CAD build for the part. Positions are in the model's coordinates, mm. A direction names the side the tool comes from. Round coordinates to 2 decimals unless told otherwise and drop trailing zeros. Write each loop counter-clockwise with the first axis right and the second up, starting at its lowest first coordinate (ties: lowest second). Pieces come first, ordered by that corner, then holes. Notation, with made-up numbers: (-1.5, 7) -> (37.5, 7) arc R25 cw to (37.5, 41) -> close; hole circle Ø7 at (89.25, -27). An arc over 180 degrees is marked (long way). Answer in a Markdown table with one row per item. Add a question column.
```python
from build123d import *

# Parameters (mm, degrees)
SKETCH1_R           = 16
SKETCH1_R_2         = 7
SKETCH1_R_3         = 1.5
BOSS_EXTRUDE1_DEPTH = 27.5
SKETCH1_3_R         = 9
SKETCH1_3_R_2       = 7
BOSS_EXTRUDE2_DEPTH = 29.5
SKETCH1_4_R         = 9
SKETCH1_4_R_2       = 7
BOSS_EXTRUDE3_DEPTH = 2


with BuildPart() as part:
    # Sketch1 → Boss-Extrude1 (new body)
    with BuildSketch(Plane.XY):
        Circle(SKETCH1_R)
        Circle(SKETCH1_R_2, mode=Mode.SUBTRACT)
        with Locations((-8.485281374, 8.485281374)):
            Circle(SKETCH1_R_3, mode=Mode.SUBTRACT)
        with Locations((8.485281374, 8.485281374)):
            Circle(SKETCH1_R_3, mode=Mode.SUBTRACT)
        with Locations((8.485281374, -8.485281374)):
            Circle(SKETCH1_R_3, mode=Mode.SUBTRACT)
        with Locations((-8.485281374, -8.485281374)):
            Circle(SKETCH1_R_3, mode=Mode.SUBTRACT)
    extrude(amount=BOSS_EXTRUDE1_DEPTH)

    # Sketch1_3 → Boss-Extrude2 (add)
    with BuildSketch(Plane.XY):
        Circle(SKETCH1_3_R)
        Circle(SKETCH1_3_R_2, mode=Mode.SUBTRACT)
    extrude(amount=BOSS_EXTRUDE2_DEPTH)

    # Sketch1_4 → Boss-Extrude3 (add)
    with BuildSketch(Plane.XY):
        Circle(SKETCH1_4_R)
        Circle(SKETCH1_4_R_2, mode=Mode.SUBTRACT)
    extrude(amount=-BOSS_EXTRUDE3_DEPTH)


solid = part.part
```
Item 1: Two-plate mould, pull along Y, no slides. Class faces 1 (the cylindrical face through (-7.68, 9.75, 13.56)), 2 (the flat face through (7, -7, 0)), 3 (the cylindrical face through (-1.172, 8.923, -0.986)): +Y half, -Y half, draft (parallel to the pull), parting line (faces both ways), or undercut.
Item 2: Saw through at C-C on y = 8. Give the cut face in (x, z).
Item 3: Saw through at B-B on x = 8.5. Give the cut face in (y, z), then the cut area to 3 significant figures.
Item 4: Saw through at A-A on y = 0. Give the cut face in (x, z), then the cut area to 3 significant figures.
Item 5: Drill centre lines: probe 1 along Y at (x, z) = (-0.5, 23); probe 2 along X at (y, z) = (9.5, 21); probe 3 along Z at (x, y) = (-10.5, -6.5). Where is each one in solid material? Low to high.
Item 6: Tool access for faces 4 (the flat face through (7, -7, 27.5)), 5 (the flat face through (0, -7.3, 29.5)): list every direction of +Z, -Z, +X, -X, +Y, -Y with a clear straight run to the whole face (end or side of a thin tool).
Item 7: Pin check, flat tips, straight feed: pin 1 (1.5 mm diameter, centred on x = 12.5, z = 7.5, fed in from +Y); pin 2 (2 mm diameter, centred on y = -8.5, z = 22.5, fed in from +X); pin 3 (1 mm diameter, centred on y = -10.5, z = 3, fed in from -X). Stop position of each tip, or through.
Recorded:
| question | item | result |
|---|---|---|
| 1 | face 1 | undercut |
| 1 | face 2 | draft |
| 1 | face 3 | parting line |
| 2 | outline | (-13.86, 0) -> (-9.9, 0) -> (-9.9, 27.5) -> (-13.86, 27.5) -> close; (-7.07, 0) -> (-4.12, 0) -> (-4.12, -2) -> (4.12, -2) -> (4.12, 0) -> (7.07, 0) -> (7.07, 27.5) -> (4.12, 27.5) -> (4.12, 29.5) -> (-4.12, 29.5) -> (-4.12, 27.5) -> (-7.07, 27.5) -> close; (9.9, 0) -> (13.86, 0) -> (13.86, 27.5) -> (9.9, 27.5) -> close |
| 3 | outline | (-13.56, 0) -> (-9.99, 0) -> (-9.99, 27.5) -> (-13.56, 27.5) -> close; (-6.99, 0) -> (-2.96, 0) -> (-2.96, -2) -> (2.96, -2) -> (2.96, 0) -> (6.99, 0) -> (6.99, 27.5) -> (2.96, 27.5) -> (2.96, 29.5) -> (-2.96, 29.5) -> (-2.96, 27.5) -> (-6.99, 27.5) -> close; (9.99, 0) -> (13.56, 0) -> (13.56, 27.5) -> (9.99, 27.5) -> close |
| 3 | area | 604 mm2 |
| 4 | outline | (-16, 0) -> (-9, 0) -> (-9, -2) -> (-7, -2) -> (-7, 29.5) -> (-9, 29.5) -> (-9, 27.5) -> (-16, 27.5) -> close; (7, -2) -> (9, -2) -> (9, 0) -> (16, 0) -> (16, 27.5) -> (9, 27.5) -> (9, 29.5) -> (7, 29.5) -> close |
| 4 | area | 511 mm2 |
| 5 | probe 1 | -15.99 to -6.98, 6.98 to 15.99 |
| 5 | probe 2 | -12.87 to -9.59, -7.38 to 7.38, 9.59 to 12.87 |
| 5 | probe 3 | 0 to 27.5 |
| 6 | face 4 | +Z |
| 6 | face 5 | +Z, +X, -X, +Y, -Y |
| 7 | pin 1 | y = 10.86 |
| 7 | pin 2 | x = 14.13 |
| 7 | pin 3 | x = -12.49 |
